from build123d import *

# Parameters (mm, degrees)
F0_R     = 12.7
F1_DEPTH = 0.8382
F3_R     = 10.1600000635
F4_DEPTH = 18.288
F5_DEPTH = 0.8382
F7_DEPTH = 0.8382


# Not quite as in the source:
# - a feature of the source that left no trace in its solid (it failed there, or was rolled back) is left out


with BuildPart() as f1:
    # F0 (on Top) → F1 (new body)
    with BuildSketch(Plane.XY):
        Circle(F0_R)
    extrude(amount=F1_DEPTH)

    # F3 (on face) → F4 (cut)
    with BuildSketch(Plane.XY.offset(0.8382)):
        Circle(F3_R)
    extrude(amount=-F4_DEPTH, mode=Mode.SUBTRACT)

    # F2 (on face) → F5 (join)
    with BuildSketch(Plane.XY.offset(0.8382)):
        with BuildLine():
            Line((-33.1810780452, -10.0371721343), (-7.7810780452, -10.0371721343))
            ThreePointArc((-7.7810780452, -10.0371721343), (-12.0158663047, 4.1120502121), (0, 12.7))
            ThreePointArc((0, 12.7), (-20.2325604445, 6.6463315632), (-33.1810780452, -10.0371721343))
        make_face()
    extrude(amount=-F5_DEPTH)

    # F6 (on face) → F7 (join)
    with BuildSketch(Plane.XY.offset(0.8382)):
        with BuildLine():
            ThreePointArc((11.5657650484, -5.2462442609), (18.062719128, 0.5983562843), (26.7811901867, 0))
            ThreePointArc((26.7811901867, 0), (14.9176093432, 9.260079703), (0.265657769, 12.6972211901))
            ThreePointArc((0.265657769, 12.6972211901), (10.7465170902, 6.7677448556), (11.5657650484, -5.2462442609))
        make_face()
    extrude(amount=-F7_DEPTH)


solid = f1.part
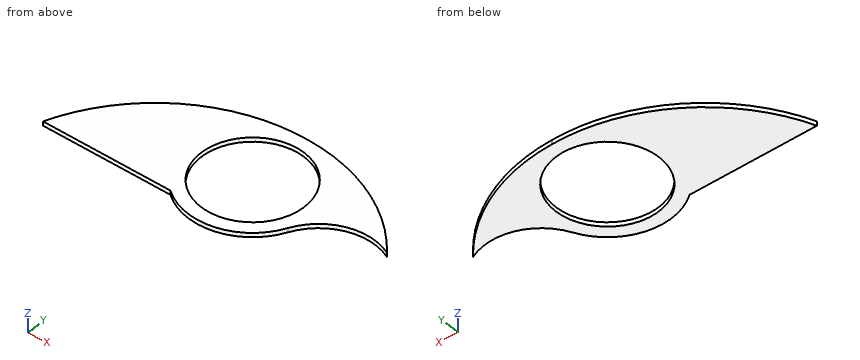
Build history of the part. All positions in model axes, mm. Coordinates: 2 decimals unless noted, no trailing zeros. Write each loop counter-clockwise with the first axis right and the second up, starting at its lowest first coordinate (ties: lowest second). Pieces come first, ordered by that corner, then holes.
(1) Cut at C-C on y = 3.5. List the corners of the cut face in (x, z).
(2) Cut at B-B on x = -6. List the corners of the cut face in (y, z), and give its area (3 significant figures).
(3) Cut at A-A on z = 0.35. List the corners of the cut face in (x, y), and give its area (3 significant figures).
(4) Pin check, flat tip, straight feed: pin 1 Ø1 at (x, y) = (-19, 8) entering from -Z. Stop position of the tip, or through.
(5) Cut at D-D on x = -16. List the corners of the cut face in (y, z), and give its area (3 significant figures).
(6) Drill centre lines: line 1 (Y direction, x = 0, z = 0.3); line 2 (Y direction, x = -0.5, z = 0.4); line 3 (X direction, y = 1.25, z = 0.3). Where is each one in solid material? Low to high.
Working result:
1. outline: (-24.17, 0) - (-9.54, 0) - (-9.54, 0.84) - (-24.17, 0.84) - close; (9.54, 0) - (23.45, 0) - (23.45, 0.84) - (9.54, 0.84) - close
2. outline: (-11.19, 0) - (-8.2, 0) - (-8.2, 0.84) - (-11.19, 0.84) - close; (8.2, 0) - (12.29, 0) - (12.29, 0.84) - (8.2, 0.84) - close
2. area: 5.94 mm2
3. outline: (-33.18, -10.04) - (-7.78, -10.04) arc R12.7 ccw to (11.57, -5.25) arc R11.21 cw to (26.78, 0) arc R35.08 ccw to (0.27, 12.7) arc R12.7 ccw to (0, 12.7) arc R34.61 ccw to start; hole circle Ø20.32 at (0, 0)
3. area: 604 mm2
4. pin 1: stops at z = 0
5. outline: (-10.04, 0) - (9.13, 0) - (9.13, 0.84) - (-10.04, 0.84) - close
5. area: 16.1 mm2
6. line 1: y = -12.7 to -10.16, 10.16 to 12.7
6. line 2: y = -12.69 to -10.15, 10.15 to 12.71
6. line 3: x = -26.39 to -10.08, 10.08 to 25.69
